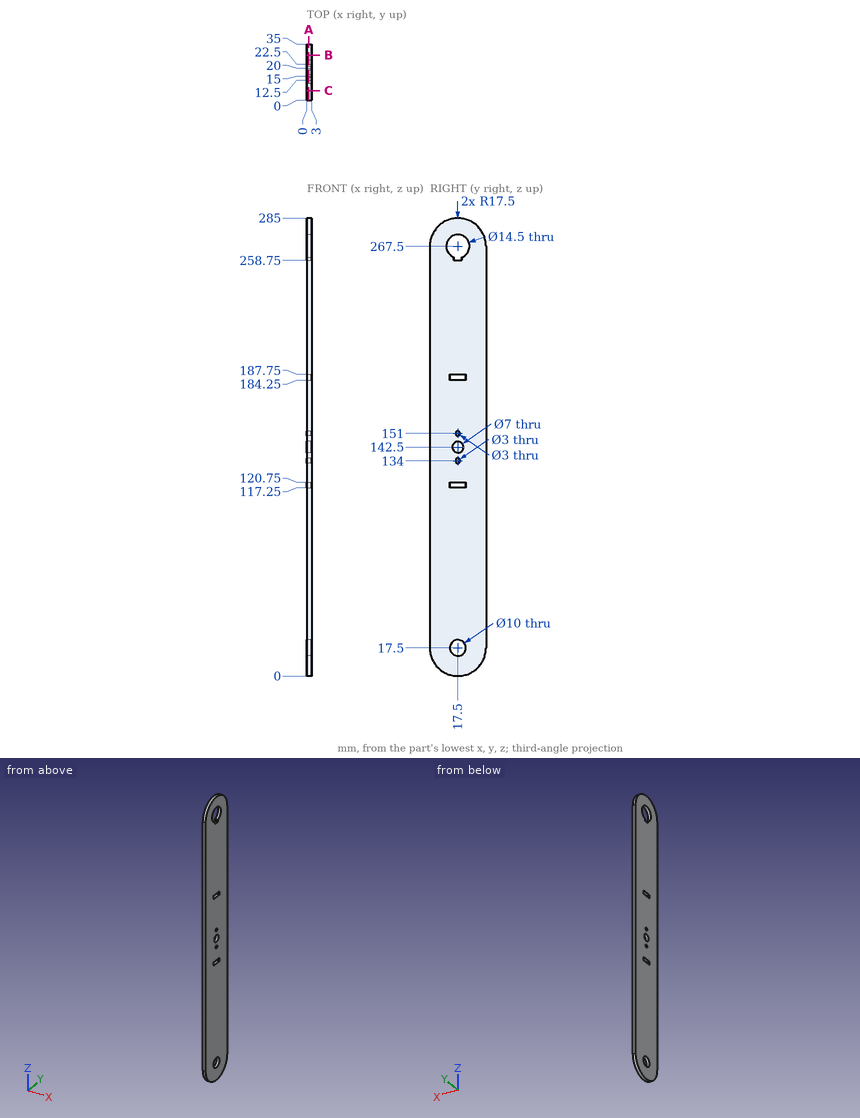
Design review of the part shown in the three views and the two pictorial views. Dimensions are in mm from the part's minimum x, y and z. Give positions to 0.01 mm unless a question says otherwise; leave off trailing zeros. Write each loop counter-clockwise with the first axis right and the second up, starting at its lowest first coordinate (ties: lowest second). Pieces come first, ordered by that corner, then holes. Notation, with made-up numbers: (38.25, -27.5) - (94.25, -27.5) arc R17 cw to (94.25, -15.5) - close; hole circle Ø6 at (-37, 15). An arc over 180 degrees is marked (long way). Return JSON: item names as keys, results as strings. Group by question number.
(1) We need section C-C, the plane y = 6. Give the boundary of the cut face in (x, z), then the cut area to 3 significant figures.
(2) We need section A-A, the plane x = 1.2. Give the boundary of the cut face in (y, z), then the cut area to 3 significant figures.
(3) We need section B-B, the plane y = 28. Give the boundary of the cut face in (x, z), then the cut area to 3 significant figures.
(4) To check wall thickness, follow probe 1 along Y at (x, z) = (0.95, 142.5); probe 2 along Z at (x, y) = (1.7, 14.5); probe 3 along Z at (x, y) = (0.9, 11.5). State the ranges of each line that lie inside material, in increasing order.
(5) Insertion check: pin 1 (1.5 mm diameter, centred on x = 2, y = 15, fed in from -Z); pin 2 (1.5 mm diameter, centred on x = 2.5, y = 21, fed in from -Z). Each pin has a flat end and moves straight along its axis. Give the tip position at first contact, or say it passes through.
Reported:
{
 "1": {"outline": "(0, 4.31) - (3, 4.31) - (3, 280.69) - (0, 280.69) - close", "area": "829 mm2"},
 "2": {"outline": "(0, 17.5) arc R17.5 ccw to (35, 17.5) - (35, 267.5) arc R17.5 ccw to (0, 267.5) - close; hole circle Ø10 at (17.5, 17.5); hole (12.5, 117.25) - (22.5, 117.25) - (22.5, 120.75) - (12.5, 120.75) - close; hole (12.5, 184.25) - (22.5, 184.25) - (22.5, 187.75) - (12.5, 187.75) - close; hole circle Ø7 at (17.5, 142.5); hole (15, 258.75) - (20, 258.75) - (20, 260.69) arc R7.25 ccw (long way) to (15, 260.69) - close; hole circle Ø3 at (17.5, 134); hole circle Ø3 at (17.5, 151)", "area": "9,340 mm2"},
 "3": {"outline": "(0, 3.5) - (3, 3.5) - (3, 281.5) - (0, 281.5) - close", "area": "834 mm2"},
 "4": {"probe 1": "y = 0 to 14, 21 to 35", "probe 2": "z = 0.26 to 13.5, 21.5 to 117.25, 120.75 to 140.7, 144.3 to 184.25, 187.75 to 260.9, 274.1 to 284.74", "probe 3": "z = 1.06 to 263.43, 271.57 to 283.94"},
 "5": {"pin 1": "stops at z = 0.09", "pin 2": "stops at z = 0.22"}
}
